For this review, take the finished solid that the model builds, in its own axes (mm). A direction names the side the tool comes from. Round coordinates to 2 decimals unless told otherwise and drop trailing zeros. Write each loop counter-clockwise with the first axis right and the second up, starting at its lowest first coordinate (ties: lowest second). Pieces come first, ordered by that corner, then holes. Notation, with made-up numbers: (24.25, 77) -> (57.25, 77) arc R23 ccw to (57.25, 112) -> close; hole circle Ø1 at (-2.5, -3.75). An arc over 180 degrees is marked (long way). Answer in a Markdown table with one row per item.
from build123d import *

# Parameters (mm, degrees)
SKETCH_1_R          = 5
EXTRUDE_1_DEPTH     = 10
EXTRUDE_2_DEPTH     = 20
SKETCH_1_4_R        = 23
SKETCH_1_4_R_2      = 15
EXTRUDE_3_DEPTH     = 45
SKETCH_1_5_R        = 17.5
SKETCH_1_5_R_2      = 15
CUT_EXTRUDE_1_DEPTH = 5
EXTRUDE_START       = 5
EXTRUDE_4_DEPTH     = 5


with BuildPart() as part:
    # Sketch 1 → Extrude 1 (new body)
    # profile 1 of 3: a face of its own
    with BuildSketch(Plane(origin=(0, 0, 0), x_dir=(1, 0, 0), z_dir=(0, 1, 0))):
        with BuildLine():
            ThreePointArc((0, -35), (35, 0), (0, 35))
            Line((0, 35), (-95, 35))
            Line((-95, 35), (-95, 17.5))
            Line((-95, 17.5), (-14.924811557, 17.5))
            ThreePointArc((-14.924811557, 17.5), (9.636631522, 20.883853402), (23, 0))
            ThreePointArc((23, 0), (9.636631522, -20.883853402), (-14.924811557, -17.5))
            Line((-14.924811557, -17.5), (-95, -17.5))
            Line((-95, -17.5), (-95, -35))
            Line((-95, -35), (0, -35))
        make_face()
    # profile 2 of 3: a face of its own
    with BuildSketch(Plane(origin=(0, 0, 0), x_dir=(1, 0, 0), z_dir=(0, 1, 0))):
        with BuildLine():
            Line((-115, -35), (-105, -35))
            Line((-105, -35), (-105, -7.5))
            Line((-105, -7.5), (-21.742814905, -7.5))
            ThreePointArc((-21.742814905, -7.5), (-22.683526432, -3.802318844), (-23, 0))
            Line((-23, 0), (-70, 0))
            Line((-70, 0), (-70, -2.5))
            Line((-70, -2.5), (-110.669872981, -2.5))
            ThreePointArc((-110.669872981, -2.5), (-116.294095226, -4.829629131), (-120, 0))
            Line((-120, 0), (-125, 0))
            Line((-125, 0), (-125, -25))
            ThreePointArc((-125, -25), (-122.071067812, -32.071067812), (-115, -35))
        make_face()
        with Locations(Location((-115, -25, 0), (0, 0, 270))):
            Circle(SKETCH_1_R, mode=Mode.SUBTRACT)
    # profile 3 of 3: a face of its own
    with BuildSketch(Plane(origin=(0, 0, 0), x_dir=(1, 0, 0), z_dir=(0, 1, 0))):
        with BuildLine():
            Line((-105, 7.5), (-105, 35))
            Line((-105, 35), (-115, 35))
            ThreePointArc((-115, 35), (-122.071067812, 32.071067812), (-125, 25))
            Line((-125, 25), (-125, 0))
            Line((-125, 0), (-120, 0))
            ThreePointArc((-120, 0), (-116.294095226, 4.829629131), (-110.669872981, 2.5))
            Line((-110.669872981, 2.5), (-70, 2.5))
            Line((-70, 2.5), (-70, 0))
            Line((-70, 0), (-23, 0))
            ThreePointArc((-23, 0), (-22.683526432, 3.802318844), (-21.742814905, 7.5))
            Line((-21.742814905, 7.5), (-105, 7.5))
        make_face()
        with Locations(Location((-115, 25, 0), (0, 0, 270))):
            Circle(SKETCH_1_R, mode=Mode.SUBTRACT)
    extrude(amount=EXTRUDE_1_DEPTH)

    # Sketch 1_3 → Extrude 2 (add)
    with BuildSketch(Plane(origin=(0, 0, 0), x_dir=(1, 0, 0), z_dir=(0, 1, 0))):
        with BuildLine():
            Line((-95, 17.5), (-95, 35))
            Line((-95, 35), (-105, 35))
            Line((-105, 35), (-105, 7.5))
            Line((-105, 7.5), (-21.742814905, 7.5))
            ThreePointArc((-21.742814905, 7.5), (-19.00338674, 12.956515443), (-14.924811557, 17.5))
            Line((-14.924811557, 17.5), (-95, 17.5))
        make_face()
        with BuildLine():
            Line((-105, -35), (-95, -35))
            Line((-95, -35), (-95, -17.5))
            Line((-95, -17.5), (-14.924811557, -17.5))
            ThreePointArc((-14.924811557, -17.5), (-19.00338674, -12.956515443), (-21.742814905, -7.5))
            Line((-21.742814905, -7.5), (-105, -7.5))
            Line((-105, -7.5), (-105, -35))
        make_face()
    extrude(amount=EXTRUDE_2_DEPTH)

    # Sketch 1_4 → Extrude 3 (add)
    with BuildSketch(Plane(origin=(0, 0, 0), x_dir=(1, 0, 0), z_dir=(0, 1, 0))):
        with Locations(Location((0, 0, 0), (0, 0, 130.459083081))):
            Circle(SKETCH_1_4_R)
        with Locations(Location((0, 0, 0), (0, 0, 90))):
            Circle(SKETCH_1_4_R_2, mode=Mode.SUBTRACT)
    extrude(amount=EXTRUDE_3_DEPTH)

    # Sketch 1_5 → Cut-Extrude 1 (cut)
    with BuildSketch(Plane(origin=(0, 0, 0), x_dir=(1, 0, 0), z_dir=(0, 1, 0))):
        with Locations(Location((0, 0, 0), (0, 0, 270))):
            Circle(SKETCH_1_5_R)
        with Locations(Location((0, 0, 0), (0, 0, 90))):
            Circle(SKETCH_1_5_R_2, mode=Mode.SUBTRACT)
    extrude(amount=CUT_EXTRUDE_1_DEPTH, mode=Mode.SUBTRACT)

    # Sketch 2 → Extrude 4 (add)
    with BuildSketch(Plane.XZ.offset(EXTRUDE_START)):
        with BuildLine():
            Line((-45, 35), (0, 35))
            ThreePointArc((0, 35), (13.228756555, 32.403703492), (24.494897428, 25))
            Line((24.494897428, 25), (-45, 25))
            Line((-45, 25), (-45, 35))
        make_face()
        with BuildLine():
            Line((-45, -25), (24.494897428, -25))
            ThreePointArc((24.494897428, -25), (13.228756555, -32.403703492), (0, -35))
            Line((0, -35), (-45, -35))
            Line((-45, -35), (-45, -25))
        make_face()
    extrude(amount=-EXTRUDE_4_DEPTH)


solid = part.part
1) Mouldability with a two-part tool opening along X and no side actions: class faces 1 (the flat face through (-45, -3, 30)), 2 (the flat face through (-71, 20, 15)), 3 (the cylindrical face through (-10.648, 2.465, -13.887)) as pulls with the +X half, pulls with the -X half, needs draft (parallel to the pull), parting line crosses it, or undercut.
Solved:
| item | result |
|---|---|
| face 1 | pulls with the -X half |
| face 2 | needs draft |
| face 3 | undercut |
2) Consider section D-D on y = 38. State the section outline as (x, z) points, then the cut area to 3 significant figures.
Solved:
| item | result |
|---|---|
| outline | circle Ø46 at (0, 0); hole circle Ø30 at (0, 0) |
| area | 955 mm² |
3) For faces 4 (the flat face through (-56, 15, 17.5)), 5 (the flat face through (-11, -3, -25)), 6 (the flat face through (-91, 5, -2.5)), list the 3-axis set-ups (+Z, -Z, +X, -X, +Y, -Y) from which the entire face can be reached by the end or side of a thin tool; tool diameter is ignored.
Solved:
| item | result |
|---|---|
| face 4 | +Z, +Y |
| face 5 | +X, -X, -Y |
| face 6 | +Y, -Y |
4) Clearance check with flat-ended pins moving along their axes: pin 1 Ø8 at (x, y) = (-53.5, 17) entering from +Z; pin 2 Ø10 at (x, z) = (-39, 22) entering from +Y; pin 3 Ø11 at (y, z) = (17, 23) entering from +X; pin 4 Ø18 at (x, z) = (0, 0) entering from +Y. State where each tip first meets the part, or that it passes through.
Solved:
| item | result |
|---|---|
| pin 1 | z = 17.5 |
| pin 2 | y = 20 |
| pin 3 | x = 14.92 |
| pin 4 | through |
5) For line 1 (X direction, y = 3, z = 0); line 2 (Z direction, x = -111, y = 5); line 3 (X direction, y = 32.5, z = 0), list the stretches that pass through material, from the lowest coordinate up. Write a range as [from, to].
Solved:
| item | result |
|---|---|
| line 1 | [-125, -120], [-70, -17.5], [17.5, 35] |
| line 2 | [-35, -28], [-22, -3], [3, 22], [28, 35] |
| line 3 | [-23, -15], [15, 23] |
6) Consider section A-A on y = 3.5. State the section outline as (x, z) points, then the cut area to 3 significant figures.
Solved:
| item | result |
|---|---|
| outline | (-125, -25) arc R10 ccw to (-115, -35) -> (0, -35) arc R35 ccw to (0, 35) -> (-115, 35) arc R10 ccw to (-125, 25) -> close; hole circle Ø10 at (-115, -25); hole circle Ø10 at (-115, 25); hole (-110.67, -2.5) -> (-70, -2.5) -> (-70, 2.5) -> (-110.67, 2.5) arc R5 ccw (long way) to start; hole circle Ø35 at (0, 0) |
| area | 9,230 mm² |
7) Consider section B-B on y = 13. State the section outline as (x, z) points, then the cut area to 3 significant figures.
Solved:
| item | result |
|---|---|
| outline | (-105, -35) -> (-95, -35) -> (-95, -17.5) -> (-14.92, -17.5) arc R23 ccw (long way) to (-14.92, 17.5) -> (-95, 17.5) -> (-95, 35) -> (-105, 35) -> (-105, 7.5) -> (-21.74, 7.5) arc R23 ccw to (-21.74, -7.5) -> (-105, -7.5) -> close; hole circle Ø30 at (0, 0) |
| area | 3,030 mm² |
8) Consider section C-C on x = -60. State the section outline as (y, z) points, then the cut area to 3 significant figures.
Solved:
| item | result |
|---|---|
| outline | (0, -35) -> (10, -35) -> (10, -17.5) -> (20, -17.5) -> (20, -7.5) -> (10, -7.5) -> (10, 7.5) -> (20, 7.5) -> (20, 17.5) -> (10, 17.5) -> (10, 35) -> (0, 35) -> close |
| area | 900 mm² |
